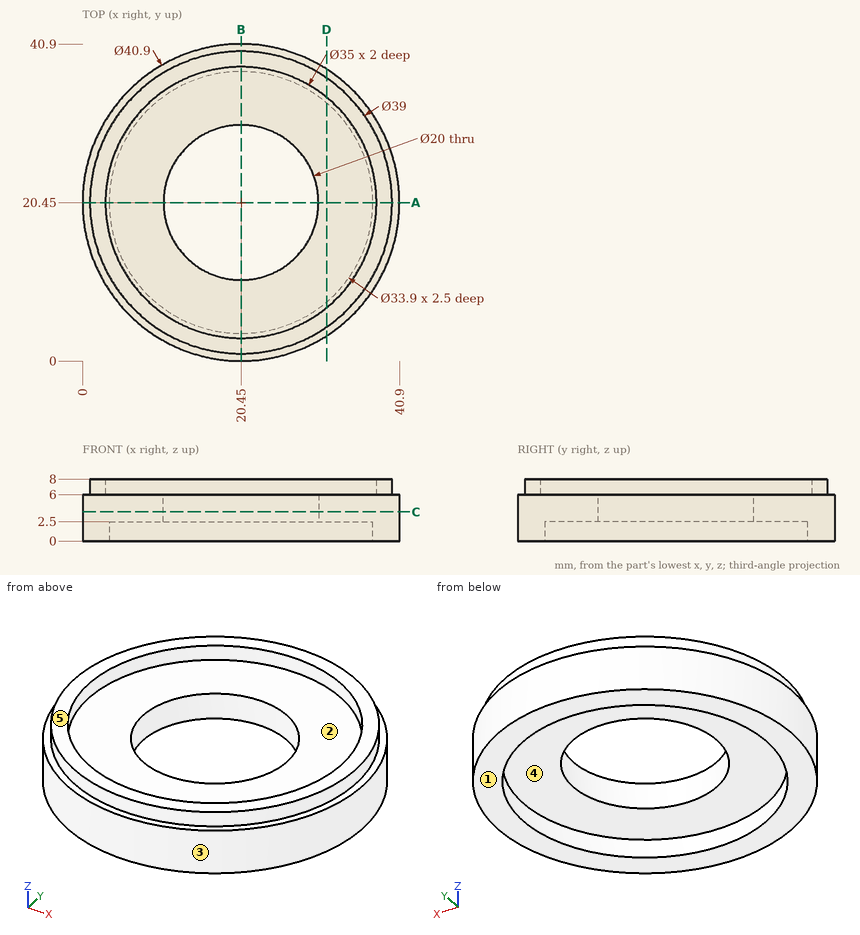
For this review, use the dimensioned drawing (mm, ordinates from the lowest corner) and the shaded views. A direction names the side the tool comes from. Round coordinates to 2 decimals unless told otherwise and drop trailing zeros. Write each loop counter-clockwise with the first axis right and the second up, starting at its lowest first coordinate (ties: lowest second). Pieces come first, ordered by that corner, then holes. Notation, with made-up numbers: M 65,50.5 L 77,50.5 A25 ccw 77,81.5 Z; hole C -28,-19 d10. An arc over 180 degrees is marked long. Use CSV: the item, a comma, the result in double quotes. Start each with the question number.
(1) We need section C-C, the plane z = 3.75. State the section outline as (x, y) points, then the cut area to 4 significant figures.
(2) The part is to be moulded in two halves that separate along X. For the marked faces 1, 2 and 3, say which applies: +X half, -X half, draft (parallel to the pull), parting line (faces both ways), or undercut.
(3) For line 1 along Y through (x, z) = (20.45, 1.7); line 2 along Y through (x, z) = (20.45, 4.5); line 3 along Z through (x, y) = (27.5, 7), list the stretches that pass through material, from the lowest coordinate up.
(4) We need section D-D, the plane x = 31.5. State the section outline as (y, z) points.
(5) Tool access review of the marked faces 4 and 5: name each direction out of +Z, -Z, +X, -X, +Y, -Y from which nothing blocks a thin tool from reaching the whole face with its end or side.
(6) Clearance check with flat-ended pins moving along their axes: P1, Ø1, axis at x = 28.5, z = 1, coming from the -Y side; P2, Ø17.5, axis at x = 19, y = 27.5, coming from the +Z side; P3, Ø12, axis at x = 17, y = 30.5, coming from the -Z side. State where each tip first meets the part, or that it passes through.
(7) We need section A-A, the plane y = 20.45. State the section outline as (x, z) points.
Findings:
1,outline,"C 20.45,20.45 d40.9; hole C 20.45,20.45 d20"
1,area,"1,000 mm^2"
2,face 1,"draft"
2,face 2,"undercut"
2,face 3,"parting line"
3,line 1,"0 to 3.5, 37.4 to 40.9"
3,line 2,"0 to 10.45, 30.45 to 40.9"
3,line 3,"2.5 to 6"
4,outline,"M 3.24,0 L 7.6,0 L 7.6,2.5 L 33.3,2.5 L 33.3,0 L 37.66,0 L 37.66,6 L 36.52,6 L 36.52,8 L 34.02,8 L 34.02,6 L 6.88,6 L 6.88,8 L 4.38,8 L 4.38,6 L 3.24,6 Z"
5,face 4,"-Z"
5,face 5,"+Z, +X, -X, +Y, -Y"
6,P1,"y = 1.44"
6,P2,"z = 6"
6,P3,"z = 2.5"
7,outline,"M 0,0 L 3.5,0 L 3.5,2.5 L 10.45,2.5 L 10.45,6 L 2.95,6 L 2.95,8 L 0.95,8 L 0.95,6 L 0,6 Z; M 30.45,2.5 L 37.4,2.5 L 37.4,0 L 40.9,0 L 40.9,6 L 39.95,6 L 39.95,8 L 37.95,8 L 37.95,6 L 30.45,6 Z"
